from build123d import *

# Parameters (mm, degrees)
SKETCH1_R           = 1.6
SKETCH1_R_2         = 2.5
BOSS_EXTRUDE1_DEPTH = 2.5
SKETCH3_R           = 2.1
BOSS_EXTRUDE2_DEPTH = 5


with BuildPart() as part:
    # Sketch1 → Boss-Extrude1 (new body)
    with BuildSketch(Plane(origin=(0, 0, 0), x_dir=(1, 0, 0), z_dir=(0, 1, 0))):
        Polygon((-8.568054712, 2.324906367), (-8.568054712, -5.675093633), (-4, -5.675093633), (-4, -9.944756554), (4, -9.944756554), (4, -5.944756554), (8.928117249, -5.944756554), (8.928117249, 2.324906367), align=None)
        with Locations((-4.568054712, -1.675093633)):
            Circle(SKETCH1_R, mode=Mode.SUBTRACT)
        with Locations((4.928117249, -1.944756554)):
            Circle(SKETCH1_R, mode=Mode.SUBTRACT)
        with Locations((0, -5.944756554)):
            Circle(SKETCH1_R_2, mode=Mode.SUBTRACT)
    extrude(amount=BOSS_EXTRUDE1_DEPTH)

    # Sketch3 → Boss-Extrude2 (add)
    with BuildSketch(Plane(origin=(0, 2.5, 0), x_dir=(1, 0, 0), z_dir=(0, 1, 0))):
        Polygon((4, -9.944756554), (-4, -9.944756554), (-4, -5.675093633), (-2.801852171, -3.446508049), (-0.938175021, -2.421485617), (1.391421416, -2.421485617), (3.297989337, -3.446508049), (4, -5.944756554), align=None)
        with Locations((0, -5.944756554)):
            Circle(SKETCH3_R, mode=Mode.SUBTRACT)
    extrude(amount=BOSS_EXTRUDE2_DEPTH)


solid = part.part
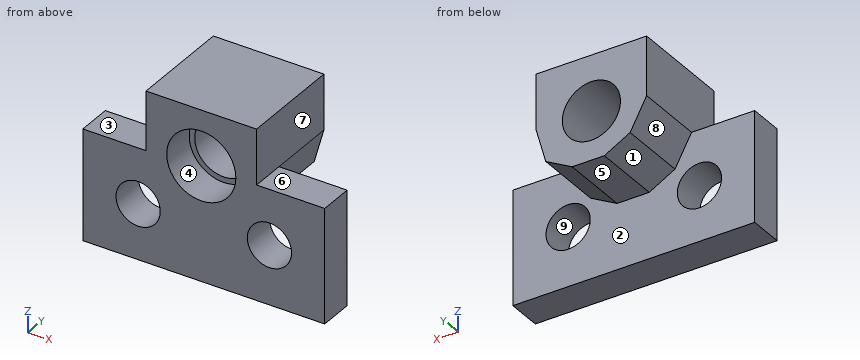
The listing builds one solid part. Answer for the finished solid, in the listing's coordinates (mm). Face numbers are marked on the shaded views. A direction names the side the tool comes from. Round coordinates to 2 decimals unless told otherwise and drop trailing zeros. Write each loop counter-clockwise with the first axis right and the second up, starting at its lowest first coordinate (ties: lowest second). Pieces come first, ordered by that corner, then holes. Notation, with made-up numbers: (6, -39.75) - (22, -39.75) arc R25 cw to (22, -15.75) - close; hole circle Ø2 at (-31, -27.75). An arc over 180 degrees is marked (long way). Use a Markdown table: item, result. Add a question column.
1. Flat-ended cylindrical pins translate along their axes: P1, Ø2, axis at x = -1.5, y = 5.5, coming from the -Z side; P2, Ø4.5, axis at y = 5.5, z = 8.5, coming from the +X side; P3, Ø1.2, axis at x = 7.5, y = 0.5, coming from the +Z side. Find the tip coordinate at first contact, or state that the pin passes through.
2. Consider line 1 (Z direction, x = 0, y = 4.5); line 2 (Z direction, x = 8, y = 0.5); line 3 (Y direction, x = 7.25, z = 3.5). Determine where each line is inside the solid, lowest interval first.
3. The part is cut by section B-B (x = 0). Write down the section's boundary in (y, z).
4. A tool of negligible diameter and unlimited length cuts with its end or side. For the marked faces 1, 2, 3, 4 and 5, from which of +Z, -Z, +X, -X, +Y, -Y can it reach the whole face along a straight path? Write none if from no direction.
5. The part is cut by section C-C (z = 7.5). Write down the section's boundary in (x, y).
6. For a pull along X with two mould halves and no side action, classify the marked faces 6, 7, 8 and 9 as +X half, -X half, draft (parallel to the pull), parting line (faces both ways), or undercut.
7. The part is cut by section A-A (y = 5.5). Write down the section's boundary in (x, z).
8. The part is cut by section D-D (x = 4.25). Write down the section's boundary in (y, z).
Reported:
| question | item | result |
|---|---|---|
| 1 | P1 | z = 2.42 |
| 1 | P2 | x = 4 |
| 1 | P3 | z = 5.94 |
| 2 | line 1 | 2.42 to 3.84, 8.04 to 9.94 |
| 2 | line 2 | -2.32 to 5.94 |
| 2 | line 3 | 0 to 2.5 |
| 3 | outline | (0, -2.32) - (2.5, -2.32) - (2.5, 2.42) - (7.5, 2.42) - (7.5, 3.84) - (2.5, 3.84) - (2.5, 3.44) - (0, 3.44) - close; (0, 8.44) - (2.5, 8.44) - (2.5, 8.04) - (7.5, 8.04) - (7.5, 9.94) - (0, 9.94) - close |
| 4 | face 1 | -Z, -X, +Y |
| 4 | face 2 | -Z, +Y |
| 4 | face 3 | +Z, -X, +Y, -Y |
| 4 | face 4 | -Y |
| 4 | face 5 | -Z, +X, -X, +Y |
| 5 | outline | (-4, 0) - (-1.96, 0) - (-1.96, 2.5) - (-1.41, 2.5) - (-1.41, 7.5) - (-4, 7.5) - close; (1.41, 2.5) - (1.96, 2.5) - (1.96, 0) - (4, 0) - (4, 7.5) - (1.41, 7.5) - close |
| 6 | face 6 | draft |
| 6 | face 7 | +X half |
| 6 | face 8 | -X half |
| 6 | face 9 | undercut |
| 7 | outline | (-4, 5.68) - (-2.8, 3.45) - (-0.94, 2.42) - (1.39, 2.42) - (3.3, 3.45) - (4, 5.94) - (4, 9.94) - (-4, 9.94) - close; hole circle Ø4.2 at (0, 5.94) |
| 8 | outline | (0, -2.32) - (2.5, -2.32) - (2.5, 0.5) - (0, 0.5) - close; (0, 3.39) - (2.5, 3.39) - (2.5, 5.94) - (0, 5.94) - close |
